The drawing under review shows one solid part. Ordinate dimensions are in mm from its lowest x, y, z. A direction names the side the tool comes from. Give positions to 0.01 mm unless a question says otherwise; leave off trailing zeros. Write each loop counter-clockwise with the first axis right and the second up, starting at its lowest first coordinate (ties: lowest second). Pieces come first, ordered by that corner, then holes. Notation, with made-up numbers: M 17,84.5 L 34,84.5 A26 ccw 34,101.5 Z; hole C 61,7.5 d3. An arc over 180 degrees is marked long. One line per item, written item: value. Start each with the question number.
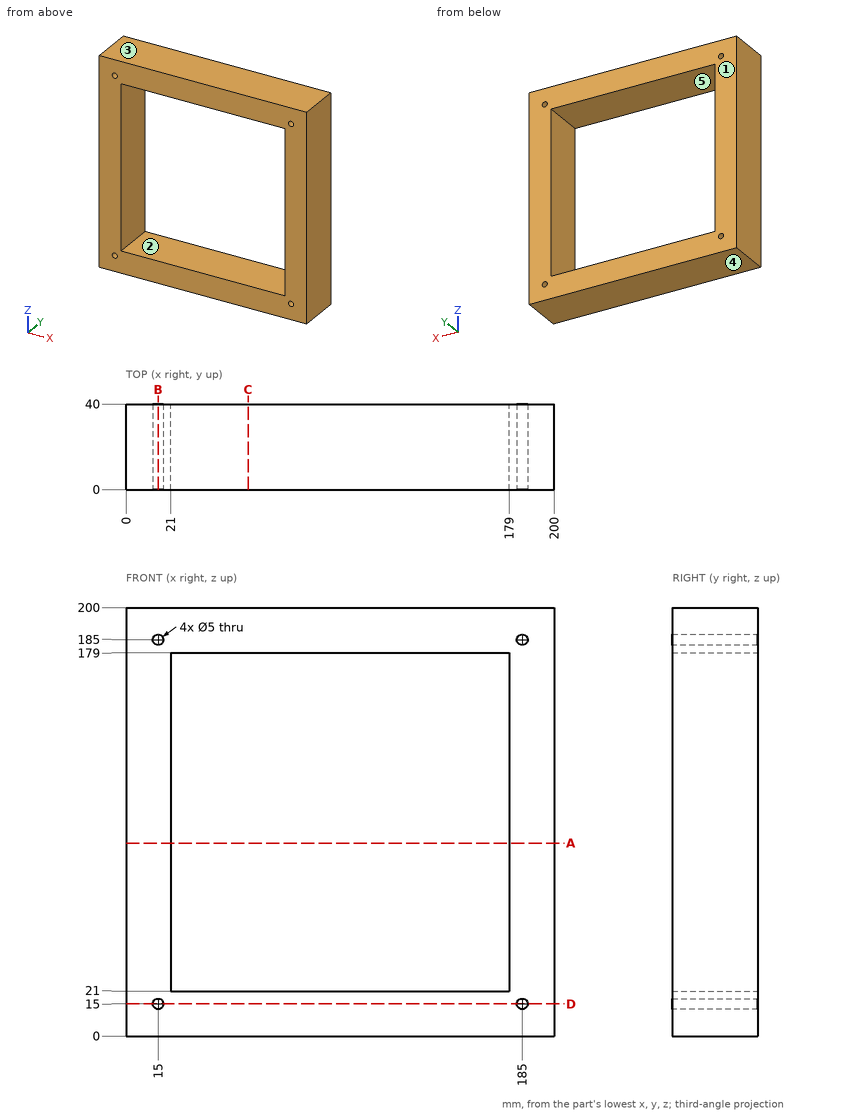
Q1. Take a section at C-C, the plane x = 57. Give the boundary of the cut face in (y, z), then the cut area to 3 significant figures.
Q2. Take a section at A-A, the plane z = 90. Give the boundary of the cut face in (x, y).
Q3. Take a section at D-D, the plane z = 15. Give the boundary of the cut face in (x, y).
Q4. Machinability: for the marked faces 4 and 5, which of the approach directions +Z, -Z, +X, -X, +Y, -Y give a long, thin tool a straight path to every point of the face, cutting with its end or side? Answer none if there is none.
Q5. Take a section at B-B, the plane x = 15. Give the boundary of the cut face in (y, z), then the cut area to 3 significant figures.
Q6. The part is to be moulded in two halves that separate along Z. For the marked faces 1, 2 and 3, say which applies: pulls with the +Z half, pulls with the -Z half, needs draft (parallel to the pull), parting line crosses it, or undercut.
Q7. Wall thickness on line 1 (X direction, y = 9, z = 185); line 2 (Z direction, x = 155, y = 36.5): over which ranges is each line inside the solid? List them lowest first. Write a range as from..to.
Results list:
1. outline: M 0,0 L 40,0 L 40,21 L 0,21 Z; M 0,179 L 40,179 L 40,200 L 0,200 Z
1. area: 1,680 mm^2
2. outline: M 0,0 L 21,0 L 21,40 L 0,40 Z; M 179,0 L 200,0 L 200,40 L 179,40 Z
3. outline: M 0,0 L 12.5,0 L 12.5,40 L 0,40 Z; M 17.5,0 L 182.5,0 L 182.5,40 L 17.5,40 Z; M 187.5,0 L 200,0 L 200,40 L 187.5,40 Z
4. face 4: -Z, +X, -X, +Y, -Y
4. face 5: +Y, -Y
5. outline: M 0,0 L 40,0 L 40,12.5 L 0,12.5 Z; M 0,17.5 L 40,17.5 L 40,182.5 L 0,182.5 Z; M 0,187.5 L 40,187.5 L 40,200 L 0,200 Z
5. area: 7,600 mm^2
6. face 1: needs draft
6. face 2: undercut
6. face 3: pulls with the +Z half
7. line 1: x = 0..12.5, 17.5..182.5, 187.5..200
7. line 2: z = 0..21, 179..200
